Autodesk Inventor part; units mm, degrees
ref_plane "YZ Plane" through (0, 0, 0) normal (1, 0, 0) x (0, 1, 0)
ref_plane "XZ Plane" through (0, 0, 0) normal (0, 1, 0) x (-1, 0, 0)
ref_plane "XY Plane" through (0, 0, 0) normal (0, 0, 1) x (1, 0, 0)
sketch "Sketch1" plane through (0, 0, 0) normal (1, 0, 0) x (0, 1, 0)
  circle A0 centre (0, 0) radius 228.6
  dimension "d0" = 457.2
extrude "Extrusion1" add sketch "Sketch1" along normal blind 12.7
hole "Hole1" at (12.7, 0, 0) direction (-1, 0, 0) diameter 25.4 end through all
sketch "Sketch3" plane through (12.7, 0, 0) normal (1, 0, 0) x (0, 0, -1)
  circle A0 centre (0, 0) radius 12.7
  point P0 (0, 215.9)
  dimension "d23" = 215.9
hole "Hole2" at (12.7, 215.9, 0) direction (-1, 0, 0) diameter 6.35 end through all
properties part number "rotator"
Geometry: final body of the model. Coordinates: model frame, mm. Round coordinates to 2 decimals unless told otherwise and drop trailing zeros. Loops run counter-clockwise (first coordinate to the right, second up) from the corner with the lowest first, then second, coordinate; pieces in that order, holes last. Notation, with made-up numbers: (-17.75, 50) -> (28.25, 50) arc R20 ccw to (28.25, 84) -> close; hole circle Ø7 at (-27.5, -30.75). An arc over 180 degrees is marked (long way). Use one line per item in the form item = value. Start each with the question number.
1) Section B-B on x = 10. Output: boundary loops of the cut face in (y, z) (3 decimals).
2) Section A-A on y = 0. Output: boundary loops of the cut face in (x, z).
3) Section C-C on z = -170. Output: boundary loops of the cut face in (x, y), then the cut area to 3 significant figures.
4) Section D-D on y = -75. Output: boundary loops of the cut face in (x, z).
5) First-contact query: P1, Ø2, axis at x = 10, z = -48.5, coming from the +Y side; P2, Ø1, axis at x = 5.5, y = -117, coming from the +Z side; P3, Ø20.5, axis at y = 0, z = 0, coming from the -X side; P4, Ø1.5, axis at x = 2, y = -125, coming from the +Z side. Flat tips, straight axial feed; report the tip coordinate or a pass-through.
6) Line query: L1, parallel to Z at x = 3.75, y = 0; L2, parallel to Y at x = 9.25, z = 8.5; L3, parallel to Z at x = 4.75, y = -132. Output: solid intervals per line, ascending.
7) Draft query along Y for faces 1 (the cylindrical face through (6.26, 12.4, 2.75)), 2 (the flat face through (0, -3, -48)), 3 (the cylindrical face through (6.26, -228.38, -10.05)). Return one class per face: released by +Y, released by -Y, zero draft, split by the parting line, or undercut.
Response:
q1.outline = circle Ø457.2 at (0, 0); hole circle Ø25.4 at (0, 0); hole circle Ø6.35 at (215.9, 0)
q2.outline = (0, -228.6) -> (12.7, -228.6) -> (12.7, -12.7) -> (0, -12.7) -> close; (0, 12.7) -> (12.7, 12.7) -> (12.7, 228.6) -> (0, 228.6) -> close
q3.outline = (0, -152.83) -> (12.7, -152.83) -> (12.7, 152.83) -> (0, 152.83) -> close
q3.area = 3,880 mm^2
q4.outline = (0, -215.95) -> (12.7, -215.95) -> (12.7, 215.95) -> (0, 215.95) -> close
q5.P1 = 223.61
q5.P2 = 196.69
q5.P3 = through
q5.P4 = 191.89
q6.L1 = -228.6 to -12.7, 12.7 to 228.6
q6.L2 = -228.44 to -9.44, 9.44 to 228.44
q6.L3 = -186.64 to 186.64
q7.face_1 = undercut
q7.face_2 = zero draft
q7.face_3 = split by the parting line
